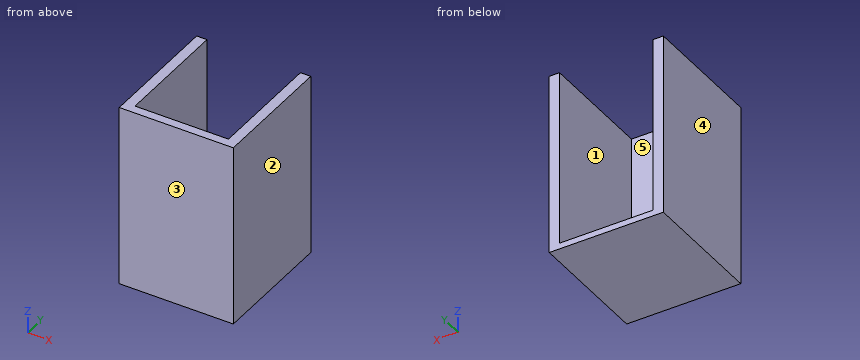
from build123d import *

# Parameters (mm, degrees)
BRKT_1_5_6_BOSS_EXTRUDE1_START       = -6
BRKT_1_5_6_BOSS_EXTRUDE1_OUTLINE_W   = 7
BRKT_1_5_6_BOSS_EXTRUDE1_OUTLINE_H   = 120
BRKT_1_5_6_BOSS_EXTRUDE1_DEPTH       = 85
BRKT_1_5_6_BOSS_EXTRUDE1_2_OUTLINE_W = 63.5
BRKT_1_5_6_BOSS_EXTRUDE1_2_OUTLINE_H = 120
BRKT_1_5_6_BOSS_EXTRUDE1_2_DEPTH     = 6
SKETCH1_W                            = 77.5
SKETCH1_H                            = 85
BOSS_EXTRUDE1_DEPTH                  = 4


# Read off the part's stored shape, not the designer's step: <BRKT_1_5_6>-<Boss-Extrude1>
with BuildPart() as part:
    # <BRKT_1_5_6>-<Boss-Extrude1> outline → <BRKT_1_5_6>-<Boss-Extrude1> (new body)
    with BuildSketch(Plane(origin=(0, 0, 0), x_dir=(1, 0, 0), z_dir=(0, 1, 0)).offset(BRKT_1_5_6_BOSS_EXTRUDE1_START)):
        with Locations((35.25, 0)):
            Rectangle(BRKT_1_5_6_BOSS_EXTRUDE1_OUTLINE_W, BRKT_1_5_6_BOSS_EXTRUDE1_OUTLINE_H)
        with Locations((-35.25, 0)):
            Rectangle(BRKT_1_5_6_BOSS_EXTRUDE1_OUTLINE_W, BRKT_1_5_6_BOSS_EXTRUDE1_OUTLINE_H)
    extrude(amount=BRKT_1_5_6_BOSS_EXTRUDE1_DEPTH)

    # BRKT_1_5_6_-_Boss-Extrude1 2 outline → BRKT_1_5_6_-_Boss-Extrude1 2 (add)
    with BuildSketch(Plane(origin=(0, 0, 0), x_dir=(1, 0, 0), z_dir=(0, 1, 0)).offset(BRKT_1_5_6_BOSS_EXTRUDE1_START)):
        Rectangle(BRKT_1_5_6_BOSS_EXTRUDE1_2_OUTLINE_W, BRKT_1_5_6_BOSS_EXTRUDE1_2_OUTLINE_H)
    extrude(amount=BRKT_1_5_6_BOSS_EXTRUDE1_2_DEPTH)

    # Sketch1 → Boss-Extrude1 (add)
    with BuildSketch(Plane(origin=(0, 0, -60), x_dir=(-1, 0, 0), z_dir=(0, 0, -1))):
        with Locations((0, 36.5)):
            Rectangle(SKETCH1_W, SKETCH1_H)
    extrude(amount=BOSS_EXTRUDE1_DEPTH)


solid = part.part
CAD build for the part. Positions are in the model's coordinates, mm. Face numbers are marked on the shaded views. A direction names the side the tool comes from. Round coordinates to 2 decimals unless told otherwise and drop trailing zeros. Order: outer loops, then holes, each group sorted by start corner. A loop starts at its lowest first (then second) coordinate and runs counter-clockwise, first axis right, second up. Notation, with made-up numbers: (78.25, 22.5) - (106.25, 22.5) arc R10 cw to (106.25, 35.5) - close; hole circle Ø4 at (-21.75, 71). An arc over 180 degrees is marked (long way). Return JSON: item names as keys, results as strings.
(1) Pin check, flat tips, straight feed: pin 1 Ø19 at (x, z) = (-10.5, -29.5) entering from +Y; pin 2 Ø19 at (x, y) = (6.5, 24.5) entering from +Z. Stop position of each tip, or through.
Answer key:
{"pin 1": "stops at y = 0", "pin 2": "stops at z = -60"}
(2) Wall check: probe 1 along X at (y, z) = (63.5, -2); probe 2 along Y at (x, z) = (11, 25); probe 3 along Z at (x, y) = (21, 13.5). Give the ranges that are in metal, low to high. Write a range as from..to.
Answer key:
{"probe 1": "x = -38.75..-31.75, 31.75..38.75", "probe 2": "y = -6..0", "probe 3": "z = -64..-60"}
(3) Cut at C-C (z = -41.5). Give the cut face in (x, y).
Answer key:
{"outline": "(-38.75, -6) - (38.75, -6) - (38.75, 79) - (31.75, 79) - (31.75, 0) - (-31.75, 0) - (-31.75, 79) - (-38.75, 79) - close"}
(4) Pull direction X, two halves, no side cores. Call the marked faces 1, 2 and 3: +X half, -X half, draft (parallel to the pull), parting line (faces both ways), or undercut.
Answer key:
{"face 1": "undercut", "face 2": "+X half", "face 3": "draft"}
(5) Cut at B-B (x = 4). Give the cut face in (y, z), then the cut area to 3 significant figures.
Answer key:
{"outline": "(-6, -64) - (79, -64) - (79, -60) - (0, -60) - (0, 60) - (-6, 60) - close", "area": "1,060 mm^2"}
(6) Tool access for the marked faces 4 and 5: list every direction of +Z, -Z, +X, -X, +Y, -Y with a clear straight run to the whole face (end or side of a thin tool).
Answer key:
{"face 4": "+Z, -Z, -X, +Y, -Y", "face 5": "+Z, +Y"}
(7) Cut at A-A (y = 45.5). Give the cut face in (x, z), then the cut area to 3 significant figures.
Answer key:
{"outline": "(-38.75, -64) - (38.75, -64) - (38.75, 60) - (31.75, 60) - (31.75, -60) - (-31.75, -60) - (-31.75, 60) - (-38.75, 60) - close", "area": "1,990 mm^2"}
